Read the model definition and answer for the solid it produces. Units are mm, in the model's axes. Give positions to 0.01 mm unless a question says otherwise; leave off trailing zeros. Order: outer loops, then holes, each group sorted by start corner. A loop starts at its lowest first (then second) coordinate and runs counter-clockwise, first axis right, second up.
```python
from build123d import *

# Parameters (mm, degrees)
BOSS_EXTRUDE1_DEPTH       = 2
F_5_0MM_DOWEL_HOLE1_D     = 5
F_5_0MM_DOWEL_HOLE1_DEPTH = 2
CUT_EXTRUDE1_REACH        = 4
SKETCH4_R                 = 2.5
CUT_EXTRUDE2_REACH        = 4


with BuildPart() as part:
    # Sketch2 → Boss-Extrude1 (new body)
    with BuildSketch(Plane(origin=(0, 0, 0), x_dir=(1, 0, 0), z_dir=(0, 1, 0))):
        with BuildLine():
            Line((100, 25), (-100, 18.75))
            ThreePointArc((-100, 18.75), (-118.75, 0), (-100, -18.75))
            Line((-100, -18.75), (100, -25))
            ThreePointArc((100, -25), (125, 0), (100, 25))
        make_face()
    extrude(amount=BOSS_EXTRUDE1_DEPTH)

    # Ø5.0mm Dowel Hole1
    with Locations(Plane(origin=(0, 2, 0), x_dir=(1, 0, 0), z_dir=(0, 1, 0))):
        with Locations((100, 0), (-100, 0)):
            Hole(F_5_0MM_DOWEL_HOLE1_D / 2, depth=F_5_0MM_DOWEL_HOLE1_DEPTH)

    # Sketch4 → Cut-Extrude1 (cut, up to next)
    with BuildSketch(Plane(origin=(0, 2, 0), x_dir=(1, 0, 0), z_dir=(0, 1, 0)), mode=Mode.PRIVATE) as cut_extrude1_sk1:
        with Locations((100, 12.2)):
            Circle(SKETCH4_R)
    cut_extrude1_tool1 = extrude(cut_extrude1_sk1.sketch, amount=-CUT_EXTRUDE1_REACH, mode=Mode.PRIVATE) & part.part
    add(cut_extrude1_tool1.solids().sort_by_distance((100, 2, -12.2))[0], mode=Mode.SUBTRACT)
    # Sketch4 → Cut-Extrude1 (cut, up to next)
    with BuildSketch(Plane(origin=(0, 2, 0), x_dir=(1, 0, 0), z_dir=(0, 1, 0)), mode=Mode.PRIVATE) as cut_extrude1_sk2:
        with Locations((100, -12.2)):
            Circle(SKETCH4_R)
    cut_extrude1_tool2 = extrude(cut_extrude1_sk2.sketch, amount=-CUT_EXTRUDE1_REACH, mode=Mode.PRIVATE) & part.part
    add(cut_extrude1_tool2.solids().sort_by_distance((100, 2, 12.2))[0], mode=Mode.SUBTRACT)
    # Sketch4 → Cut-Extrude1 (cut, up to next)
    with BuildSketch(Plane(origin=(0, 2, 0), x_dir=(1, 0, 0), z_dir=(0, 1, 0)), mode=Mode.PRIVATE) as cut_extrude1_sk3:
        with Locations((112.2, 0)):
            Circle(SKETCH4_R)
    cut_extrude1_tool3 = extrude(cut_extrude1_sk3.sketch, amount=-CUT_EXTRUDE1_REACH, mode=Mode.PRIVATE) & part.part
    add(cut_extrude1_tool3.solids().sort_by_distance((112.2, 2, 0))[0], mode=Mode.SUBTRACT)
    # Sketch4 → Cut-Extrude1 (cut, up to next)
    with BuildSketch(Plane(origin=(0, 2, 0), x_dir=(1, 0, 0), z_dir=(0, 1, 0)), mode=Mode.PRIVATE) as cut_extrude1_sk4:
        with Locations((87.8, 0)):
            Circle(SKETCH4_R)
    cut_extrude1_tool4 = extrude(cut_extrude1_sk4.sketch, amount=-CUT_EXTRUDE1_REACH, mode=Mode.PRIVATE) & part.part
    add(cut_extrude1_tool4.solids().sort_by_distance((87.8, 2, 0))[0], mode=Mode.SUBTRACT)
    # Sketch4 → Cut-Extrude1 (cut, up to next)
    with BuildSketch(Plane(origin=(0, 2, 0), x_dir=(1, 0, 0), z_dir=(0, 1, 0)), mode=Mode.PRIVATE) as cut_extrude1_sk5:
        with Locations((-100, 12.2)):
            Circle(SKETCH4_R)
    cut_extrude1_tool5 = extrude(cut_extrude1_sk5.sketch, amount=-CUT_EXTRUDE1_REACH, mode=Mode.PRIVATE) & part.part
    add(cut_extrude1_tool5.solids().sort_by_distance((-100, 2, -12.2))[0], mode=Mode.SUBTRACT)
    # Sketch4 → Cut-Extrude1 (cut, up to next)
    with BuildSketch(Plane(origin=(0, 2, 0), x_dir=(1, 0, 0), z_dir=(0, 1, 0)), mode=Mode.PRIVATE) as cut_extrude1_sk6:
        with Locations((-87.8, 0)):
            Circle(SKETCH4_R)
    cut_extrude1_tool6 = extrude(cut_extrude1_sk6.sketch, amount=-CUT_EXTRUDE1_REACH, mode=Mode.PRIVATE) & part.part
    add(cut_extrude1_tool6.solids().sort_by_distance((-87.8, 2, 0))[0], mode=Mode.SUBTRACT)
    # Sketch4 → Cut-Extrude1 (cut, up to next)
    with BuildSketch(Plane(origin=(0, 2, 0), x_dir=(1, 0, 0), z_dir=(0, 1, 0)), mode=Mode.PRIVATE) as cut_extrude1_sk7:
        with Locations((-112.2, 0)):
            Circle(SKETCH4_R)
    cut_extrude1_tool7 = extrude(cut_extrude1_sk7.sketch, amount=-CUT_EXTRUDE1_REACH, mode=Mode.PRIVATE) & part.part
    add(cut_extrude1_tool7.solids().sort_by_distance((-112.2, 2, 0))[0], mode=Mode.SUBTRACT)
    # Sketch4 → Cut-Extrude1 (cut, up to next)
    with BuildSketch(Plane(origin=(0, 2, 0), x_dir=(1, 0, 0), z_dir=(0, 1, 0)), mode=Mode.PRIVATE) as cut_extrude1_sk8:
        with Locations((-100, -12.2)):
            Circle(SKETCH4_R)
    cut_extrude1_tool8 = extrude(cut_extrude1_sk8.sketch, amount=-CUT_EXTRUDE1_REACH, mode=Mode.PRIVATE) & part.part
    add(cut_extrude1_tool8.solids().sort_by_distance((-100, 2, 12.2))[0], mode=Mode.SUBTRACT)

    # Sketch16 → Cut-Extrude2 (cut, up to next)
    with BuildSketch(Plane(origin=(0, 2, 0), x_dir=(1, 0, 0), z_dir=(0, 1, 0)), mode=Mode.PRIVATE) as cut_extrude2_sk1:
        with BuildLine():
            Line((-50, -2.5), (50, -2.5))
            ThreePointArc((50, -2.5), (52.5, 0), (50, 2.5))
            Line((50, 2.5), (-50, 2.5))
            ThreePointArc((-50, 2.5), (-52.5, 0), (-50, -2.5))
        make_face()
    cut_extrude2_tool1 = extrude(cut_extrude2_sk1.sketch, amount=-CUT_EXTRUDE2_REACH, mode=Mode.PRIVATE) & part.part
    add(cut_extrude2_tool1.solids().sort_by_distance((0, 2, 0))[0], mode=Mode.SUBTRACT)


solid = part.part
```
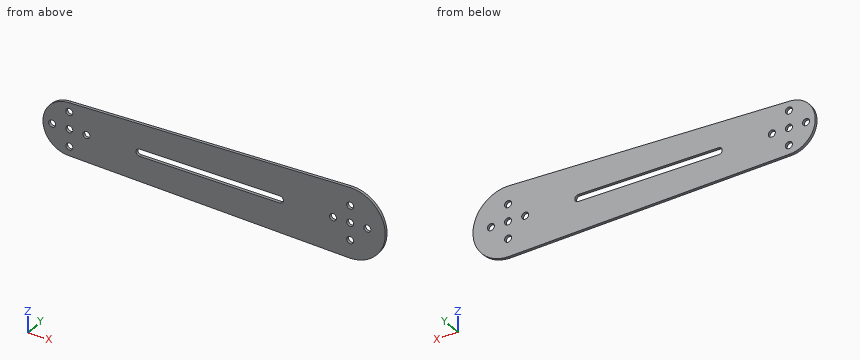
1) The part is cut by section C-C on x = 112.2. Determine the outline of the cut face in (y, z).
Final values:
outline: (0, -21.82) - (2, -21.82) - (2, -2.5) - (0, -2.5) - close; (0, 2.5) - (2, 2.5) - (2, 21.82) - (0, 21.82) - close
2) Consider L1, parallel to Z at x = 100, y = 0.55; L2, parallel to X at y = 1.3, z = 12.2; L3, parallel to Z at x = -26.5, y = 0.4. Determine where each line is inside the solid, lowest interval first.
Final values:
L1: z = -25 to -14.7, -9.7 to -2.5, 2.5 to 9.7, 14.7 to 25
L2: x = -114.24 to -102.5, -97.5 to 97.5, 102.5 to 121.82
L3: z = -21.05 to -2.5, 2.5 to 21.05
3) The part is cut by section A-A on y = 1.45. Count the separate pieces of the cut face and the enclosed holes in it, and give its area (3 significant figures).
Final values:
separate pieces: 1
enclosed holes: 11
area: 9,570 mm2
4) The part is cut by section D-D on z = 12.2. Determine the outline of the cut face in (x, y).
Final values:
outline: (-114.24, 0) - (-102.5, 0) - (-102.5, 2) - (-114.24, 2) - close; (-97.5, 0) - (97.5, 0) - (97.5, 2) - (-97.5, 2) - close; (102.5, 0) - (121.82, 0) - (121.82, 2) - (102.5, 2) - close
5) Given pin 1 (4 mm diameter, centred on x = -100, z = -12.2, fed in from -Y), flat-ended and moving along its own axis, determine where the tip first touches the part or whether it passes through.
Final values:
pin 1: passes through
